Job drawing, mm, ordinate dimensions from the low corner. One solid piece. Round coordinates to 2 decimals unless told otherwise and drop trailing zeros. Loops run counter-clockwise (first coordinate to the right, second up) from the corner with the lowest first, then second, coordinate; pieces in that order, holes last.
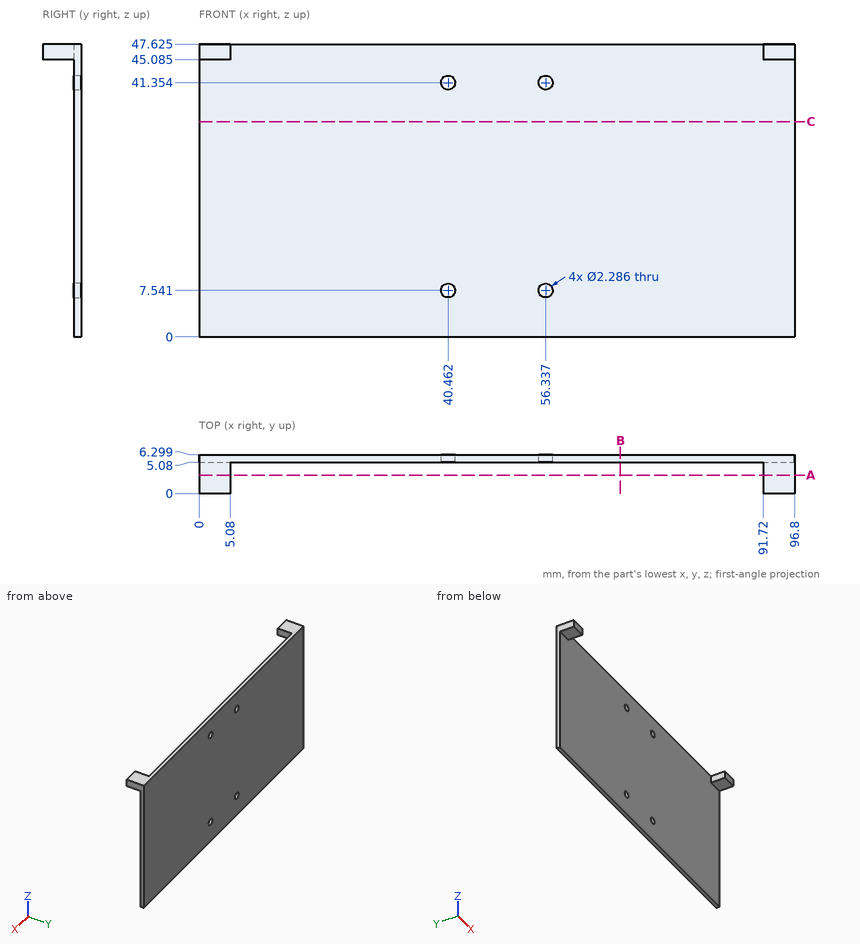
Item 1: Cut at A-A, the plane y = 3. Give the cut face in (x, z) (1 decimal).
Answers follow:
outline: (0, 45.1) - (5.1, 45.1) - (5.1, 47.6) - (0, 47.6) - close; (91.7, 45.1) - (96.8, 45.1) - (96.8, 47.6) - (91.7, 47.6) - close
Item 2: Cut at C-C, the plane z = 35. Give the cut face in (x, y).
Answers follow:
outline: (0, 5.08) - (96.8, 5.08) - (96.8, 6.3) - (0, 6.3) - close
Item 3: Probe line 1 (Y direction, x = 43, z = 24); line 2 (X direction, y = 5.25, z = 8) (1 decimal). List the from-to ranges inside material, lowest first.
Answers follow:
line 1: y = 5.08 to 6.3
line 2: x = 0 to 39.4, 41.5 to 55.3, 57.4 to 96.8
Item 4: Cut at B-B, the plane x = 68.5. Give the cut face in (y, z) (1 decimal).
Answers follow:
outline: (5.1, 0) - (6.3, 0) - (6.3, 47.6) - (5.1, 47.6) - close
Item 5: Flat gauge pins, fed straight in: P1, Ø2.5, axis at x = 2.5, y = 2.5, coming from the -Z side (1 decimal); P2, Ø1, axis at y = 5, z = 36, coming from the +X side; P3, Ø6, axis at x = 22, z = 16, coming from the -Y side; P4, Ø1.4, axis at x = 56.34, z = 7.54, coming from the +Y side. Where does each tip first touch, or does it go through?
Answers follow:
P1: stops at z = 45.1
P2: stops at x = 96.8
P3: stops at y = 5.08
P4: passes through
